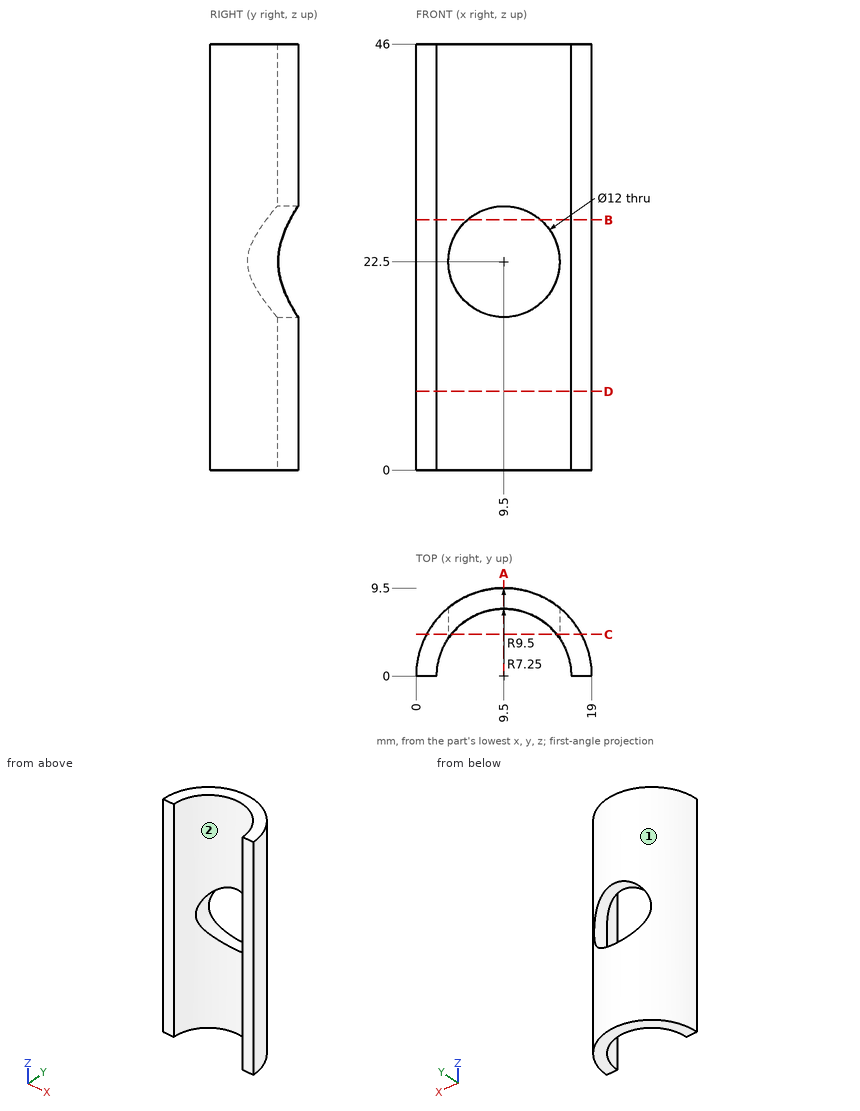
Answer from the drawing. Dimensions are ordinates in mm from the lowest x, y and z of the part. Round coordinates to 2 decimals unless told otherwise and drop trailing zeros. Write each loop counter-clockwise with the first axis right and the second up, starting at its lowest first coordinate (ties: lowest second). Pieces come first, ordered by that corner, then holes. Notation, with made-up numbers: (79.5, 49.25) -> (110.5, 49.25) arc R29 cw to (110.5, 86.25) -> close; hole circle Ø3 at (-1, 64). An arc over 180 degrees is marked (long way). Write each question's results on one line, items separated by ' | '.
1) The part is cut by section B-B (z = 27). Write down the section's boundary in (x, y).
Findings:
outline: (0, 0) -> (2.25, 0) arc R7.25 cw to (5.53, 6.07) -> (5.53, 8.63) arc R9.5 ccw to start; (13.47, 6.07) arc R7.25 cw to (16.75, 0) -> (19, 0) arc R9.5 ccw to (13.47, 8.63) -> close
2) The part is cut by section A-A (x = 9.5). Write down the section's boundary in (y, z), and give its area (3 significant figures).
Findings:
outline: (7.25, 0) -> (9.5, 0) -> (9.5, 16.5) -> (7.25, 16.5) -> close; (7.25, 28.5) -> (9.5, 28.5) -> (9.5, 46) -> (7.25, 46) -> close | area: 76.5 mm²
3) Consider line 1 along X through (y, z) = (6.1, 22.5); line 2 along X through (y, z) = (2, 10.5); line 3 along Y through (x, z) = (9.5, 38.5). Determine where each line is inside the solid, lowest interval first. Write a range as [from, to].
Findings:
line 1: x = [2.22, 3.5], [15.5, 16.78] | line 2: x = [0.21, 2.53], [16.47, 18.79] | line 3: y = [7.25, 9.5]
4) The part is cut by section C-C (y = 4.5). Write down the section's boundary in (x, z).
Findings:
outline: (1.13, 0) -> (3.82, 0) -> (3.82, 20.58) arc R6 cw to (3.82, 24.42) -> (3.82, 46) -> (1.13, 46) -> close; (15.18, 0) -> (17.87, 0) -> (17.87, 46) -> (15.18, 46) -> (15.18, 24.42) arc R6 cw to (15.18, 20.58) -> close
5) For a pull along X with two mould halves and no side action, classify the marked faces 1 and 2 as +X half, -X half, draft (parallel to the pull), parting line (faces both ways), or undercut.
Findings:
face 1: parting line | face 2: undercut
6) Flat-ended cylindrical pins translate along their axes: pin 1 (1.5 mm diameter, centred on y = 3.5, z = 12.5, fed in from -X); pin 2 (9.5 mm diameter, centred on x = 9.5, z = 22.5, fed in from -Y). Find the tip coordinate at first contact, or state that the pin passes through.
Findings:
pin 1: stops at x = 0.41 | pin 2: passes through
7) The part is cut by section D-D (z = 8.5). Write down the section's boundary in (x, y).
Findings:
outline: (0, 0) -> (2.25, 0) arc R7.25 cw to (16.75, 0) -> (19, 0) arc R9.5 ccw to start
